The model under review builds one solid part; all positions refer to its coordinate system, in mm. Face numbers are marked on the shaded views. A direction names the side the tool comes from. Round coordinates to 2 decimals unless told otherwise and drop trailing zeros. Loops run counter-clockwise (first coordinate to the right, second up) from the corner with the lowest first, then second, coordinate; pieces in that order, holes last. Notation, with made-up numbers: M 75,-27 L 88,-27 A19 cw 88,-13 Z; hole C 89.25,-20.75 d5. An arc over 180 degrees is marked long. One line per question, with ' | ' between items.
from build123d import *

# Parameters (mm, degrees)
F1_DEPTH = 25
F3_DEPTH = 25


with BuildPart() as f1:
    # F0 (on Top) → F1 (new body)
    with BuildSketch(Plane.XY):
        Polygon((-22.048956, -2.44946), (-22.048956, 0.05054), (-27.048956, 0.05054), (-27.048956, -6.949464), (-22.048956, -6.949464), (-22.048956, -4.449464), (2.951044, -4.449464), (2.951044, 35.550536), (-22.048956, 35.550536), (-22.048956, 38.050536), (-27.048956, 38.050536), (-27.048956, 30.050536), (-22.048956, 30.050536), (-22.048956, 32.550536), (-0.048956, 32.550536), (-0.048956, -2.44946), align=None)
    extrude(amount=F1_DEPTH)

    # F2 (on Right) → F3 (cut)
    with BuildSketch(Plane.YZ):
        with BuildLine():
            Line((18.382891, 6), (18.382891, 19))
            ThreePointArc((18.382891, 19), (15.382891, 22), (12.382891, 19))
            Line((12.382891, 19), (12.382891, 6))
            ThreePointArc((12.382891, 6), (15.382891, 3), (18.382891, 6))
        make_face()
    extrude(amount=F3_DEPTH, mode=Mode.SUBTRACT)


solid = f1.part
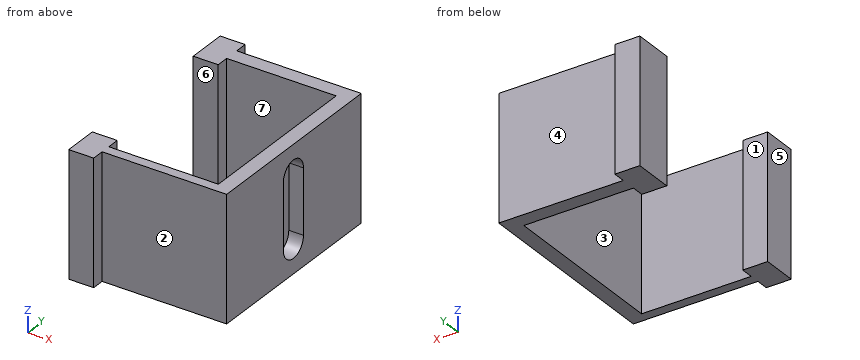
1) Insertion check: P1, Ø2, axis at x = -9, z = 16.5, coming from the +Y side; P2, Ø1.5, axis at x = -0.5, y = 0, coming from the -Z side; P3, Ø1.5, axis at x = 1, z = 11.5, coming from the -Y side; P4, Ø3, axis at y = 15.5, z = 15.5, coming from the +X side. Each pin has a flat end and moves straight along its axis. Give the tip position at first contact, or say it passes through.
Output values:
P1: stops at y = 35.55 | P2: stops at z = 0 | P3: stops at y = -4.45 | P4: stops at x = 0
2) Add section B-B on z = 17.75. State the section outline as (x, y) points.
Output values:
outline: M -27.05,-6.95 L -22.05,-6.95 L -22.05,-4.45 L 2.95,-4.45 L 2.95,12.38 L 0,12.38 L 0,18.38 L 2.95,18.38 L 2.95,35.55 L -22.05,35.55 L -22.05,38.05 L -27.05,38.05 L -27.05,30.05 L -22.05,30.05 L -22.05,32.55 L -0.05,32.55 L -0.05,-2.45 L -22.05,-2.45 L -22.05,0.05 L -27.05,0.05 Z
3) Add section C-C on x = -15. State the section outline as (y, z) points.
Output values:
outline: M -4.45,0 L -2.45,0 L -2.45,25 L -4.45,25 Z; M 32.55,0 L 35.55,0 L 35.55,25 L 32.55,25 Z
4) Machinability: for the marked faces 1, 2, 3 and 4, which of the approach directions +Z, -Z, +X, -X, +Y, -Y give a long, thin tool a straight path to every point of the face, cutting with its end or side? Answer none if there is none.
Output values:
face 1: +Z, -Z, -X | face 2: +Z, -Z, +X, -Y | face 3: +Z, -Z | face 4: +Z, -Z, +X, +Y
5) Add section A-A on y = -1. State the section outline as (x, z) points, then the cut area to 3 significant figures.
Output values:
outline: M -27.05,0 L -22.05,0 L -22.05,25 L -27.05,25 Z; M -0.05,0 L 2.95,0 L 2.95,25 L -0.05,25 Z | area: 200 mm²
6) For line 1 (Y direction, x = -5, z = 19.25); line 2 (Y direction, x = 1, z = 10); line 3 (X direction, y = 20, z = 5), list the stretches that pass through material, from the lowest coordinate up.
Output values:
line 1: y = -4.45 to -2.45, 32.55 to 35.55 | line 2: y = -4.45 to 12.38, 18.38 to 35.55 | line 3: x = -0.05 to 2.95
7) Add section D-D on y = 5. State the section outline as (x, z) points, then the cut area to 3 significant figures.
Output values:
outline: M -0.05,0 L 2.95,0 L 2.95,25 L -0.05,25 Z | area: 75.0 mm²
8) Mouldability with a two-part tool opening along X and no side actions: class the marked faces 5, 6 and 7 as +X half, -X half, draft (parallel to the pull), parting line (faces both ways), or undercut.
Output values:
face 5: -X half | face 6: draft | face 7: undercut
